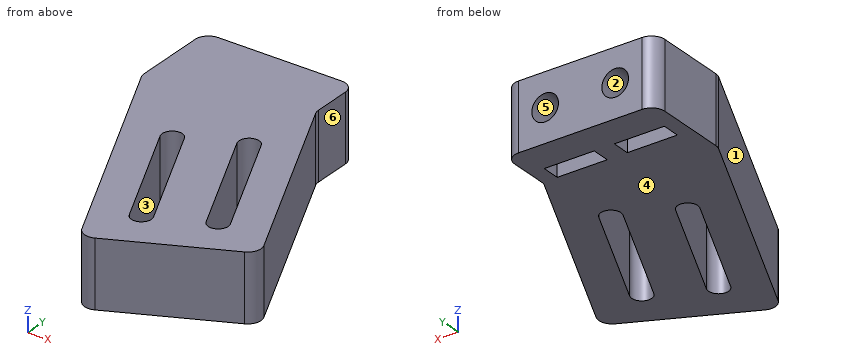
from build123d import *

# Parameters (mm, degrees)
BOSS_EXTRUDE1_DEPTH          = 10
F_4_0_4_DIAMETER_HOLE1_D     = 4
F_4_0_4_DIAMETER_HOLE1_DEPTH = 15
F_4_0_4_DIAMETER_HOLE1_TIP   = 1.201721238
SKETCH6_W                    = 7.5
SKETCH6_H                    = 2.7
CUT_EXTRUDE1_DEPTH           = 8.75
FILLET1_R                    = 2


with BuildPart() as part:
    # Sketch1 → Boss-Extrude1 (new body)
    with BuildSketch(Plane.XY):
        Polygon((0, 0), (22.5, 0), (22.5, -8), (37.747058824, -40.611764706), (17.364705882, -50.141176471), (0, -13), align=None)
        with BuildLine():
            Line((13.388235294, -22.747058824), (21.858823529, -40.864705882))
            ThreePointArc((21.858823529, -40.864705882), (21.135294118, -42.858823529), (19.141176471, -42.135294118))
            Line((19.141176471, -42.135294118), (10.670588235, -24.017647059))
            ThreePointArc((10.670588235, -24.017647059), (11.394117647, -22.023529412), (13.388235294, -22.747058824))
        make_face(mode=Mode.SUBTRACT)
        with BuildLine():
            Line((21.994117647, -18.723529412), (30.464705882, -36.841176471))
            ThreePointArc((30.464705882, -36.841176471), (29.741176471, -38.835294118), (27.747058824, -38.111764706))
            Line((27.747058824, -38.111764706), (19.276470588, -19.994117647))
            ThreePointArc((19.276470588, -19.994117647), (20, -18), (21.994117647, -18.723529412))
        make_face(mode=Mode.SUBTRACT)
    extrude(amount=BOSS_EXTRUDE1_DEPTH)

    # Ø4.0 (4) Diameter Hole1
    with Locations(Plane(origin=(0, 0, 0), x_dir=(1, 0, 0), z_dir=(0, 1, 0))):
        with Locations((6, -5), (16.5, -5)):
            Hole(F_4_0_4_DIAMETER_HOLE1_D / 2, depth=F_4_0_4_DIAMETER_HOLE1_DEPTH)
            with Locations((0, 0, -(F_4_0_4_DIAMETER_HOLE1_DEPTH + F_4_0_4_DIAMETER_HOLE1_TIP / 2))):  # 118° drill point
                Cone(0, F_4_0_4_DIAMETER_HOLE1_D / 2, F_4_0_4_DIAMETER_HOLE1_TIP, mode=Mode.SUBTRACT)

    # Sketch6 → Cut-Extrude1 (cut)
    with BuildSketch(Plane.XY):
        with Locations((6, -6.35)):
            Rectangle(SKETCH6_W, SKETCH6_H)
        with Locations((16.5, -6.35)):
            Rectangle(SKETCH6_W, SKETCH6_H)
    extrude(amount=CUT_EXTRUDE1_DEPTH, mode=Mode.SUBTRACT)

    # Fillet1
    fillet1_edges = [part.edges().sort_by_distance(p)[0] for p in [
        (0, 0, 5),
        (22.5, 0, 5),
        (22.5, -8, 5),
        (37.747058824, -40.611764706, 5),
        (17.364705882, -50.141176471, 5),
        (0, -13, 5),
    ]]
    fillet(fillet1_edges, radius=FILLET1_R)


solid = part.part
The listing builds one solid part. Answer for the finished solid, in the listing's coordinates (mm). Face numbers are marked on the shaded views. A direction names the side the tool comes from. Coordinates: 2 decimals unless noted, no trailing zeros. Loops run counter-clockwise (first coordinate to the right, second up) from the corner with the lowest first, then second, coordinate; pieces in that order, holes last.
1) Find section D-D on x = 24.5. Write down the section's boundary in (y, z), then the cut area to 3 significant figures.
2) Flat-ended cylindrical pins translate along their axes: pin 1 Ø0.8 at (y, z) = (-7, 5) entering from +X; pin 2 Ø3 at (x, z) = (16.5, 5) entering from +Y; pin 3 Ø4.5 at (x, z) = (6, 5) entering from -Y. Find the tip coordinate at first contact, or state that the pin passes through.
3) Find the intervals of material crossed by L1, parallel to Z at x = 16.5, y = -2.6; L2, parallel to X at y = -29, z = 8.75; L3, parallel to X at y = -36.5, z = 3.75, in increasing order.
4) Find section C-C on x = 9. Write down the section's boundary in (y, z).
5) Find section A-A on z = 7.75. Write down the section's boundary in (x, y).
6) Determine the mould class of the marked faces 4, 5 and 6 for opening direction Z: pulls with the +Z half, pulls with the -Z half, needs draft (parallel to the pull), parting line crosses it, or undercut.
7) A tool of negligible diameter and unlimited length cuts with its end or side. For the marked faces 1, 2 and 3, from which of +Z, -Z, +X, -X, +Y, -Y can it reach the whole face along a straight path? Write none if from no direction.
8) Find section B-B on y = -32.5. Write down the section's boundary in (x, z), then the cut area to 3 significant figures.
Values:
1. outline: (-46.81, 0) - (-31.17, 0) - (-31.17, 10) - (-46.81, 10) - close; (-24.08, 0) - (-12.28, 0) - (-12.28, 10) - (-24.08, 10) - close
1. area: 274 mm2
2. pin 1: stops at x = 22.5
2. pin 2: stops at y = -15.3
2. pin 3: stops at y = -30.65
3. L1: z = 0 to 3, 7 to 10
3. L2: x = 7.48 to 13, 16.31 to 23.49, 26.8 to 32.32
3. L3: x = 10.99 to 16.51, 19.82 to 26.99, 30.31 to 35.82
4. outline: (-32.25, 0) - (-7.7, 0) - (-7.7, 8.75) - (-5, 8.75) - (-5, 0) - (0, 0) - (0, 10) - (-32.25, 10) - close
5. outline: (0, -12.56) arc R2 ccw to (0.19, -13.4) - (16.52, -48.33) arc R2 ccw to (19.18, -49.29) - (35.94, -41.46) arc R2 ccw to (36.9, -38.8) - (22.69, -8.4) arc R2 cw to (22.5, -7.56) - (22.5, -2) arc R2 ccw to (20.5, 0) - (2, 0) arc R2 ccw to (0, -2) - close; hole (2.25, -7.7) - (9.75, -7.7) - (9.75, -5) - (2.25, -5) - close; hole (10.67, -24.02) - (19.14, -42.14) arc R1.5 ccw to (21.86, -40.86) - (13.39, -22.75) arc R1.5 ccw to start; hole (12.75, -7.7) - (20.25, -7.7) - (20.25, -5) - (12.75, -5) - close; hole (19.28, -19.99) - (27.75, -38.11) arc R1.5 ccw to (30.46, -36.84) - (21.99, -18.72) arc R1.5 ccw to start
6. face 4: pulls with the -Z half
6. face 5: undercut
6. face 6: needs draft
7. face 1: +Z, -Z, -X, -Y
7. face 2: +Y
7. face 3: +Z, -Z
8. outline: (9.12, 0) - (14.64, 0) - (14.64, 10) - (9.12, 10) - close; (17.95, 0) - (25.12, 0) - (25.12, 10) - (17.95, 10) - close; (28.44, 0) - (33.95, 0) - (33.95, 10) - (28.44, 10) - close
8. area: 182 mm2
